Design review of the part built by this model. Coordinates are the model's own, in mm. Face numbers are marked on the shaded views. A direction names the side the tool comes from. Round coordinates to 2 decimals unless told otherwise and drop trailing zeros. Loops run counter-clockwise (first coordinate to the right, second up) from the corner with the lowest first, then second, coordinate; pieces in that order, holes last. Notation, with made-up numbers: (-14.75, 53.25) -> (32.25, 53.25) arc R27 cw to (32.25, 77.25) -> close; hole circle Ø1 at (-31, 27). An arc over 180 degrees is marked (long way). Answer as CSV lines item,"result". Start each with the question number.
```python
from build123d import *

# Parameters (mm, degrees)
F1_DEPTH = 10
F2_W     = 30
F2_H     = 30
F3_DEPTH = 28.5
F4_R     = 10.5
F5_DEPTH = 57.001


with BuildPart() as f1:
    # F0 (on Top) → F1 (new body, symmetric)
    with BuildSketch(Plane.XY):
        Polygon((-12.5, -25), (12.5, -25), (12.5, 25), (-12.5, 25), (-12.5, 15), (-54.5, 15), (-54.5, -15), (-12.5, -15), align=None)
    extrude(amount=F1_DEPTH, both=True)

    # F2 (on Top) → F3 (join, symmetric)
    with BuildSketch(Plane.XY):
        with Locations((-39.5, 0)):
            Rectangle(F2_W, F2_H)
    extrude(amount=F3_DEPTH, both=True)

    # F4 (on face) → F5 (cut, through all)
    with BuildSketch(Plane.XY.offset(28.5)):
        with Locations((-39.5, 0)):
            Circle(F4_R)
    extrude(amount=-F5_DEPTH, mode=Mode.SUBTRACT)


solid = f1.part
```
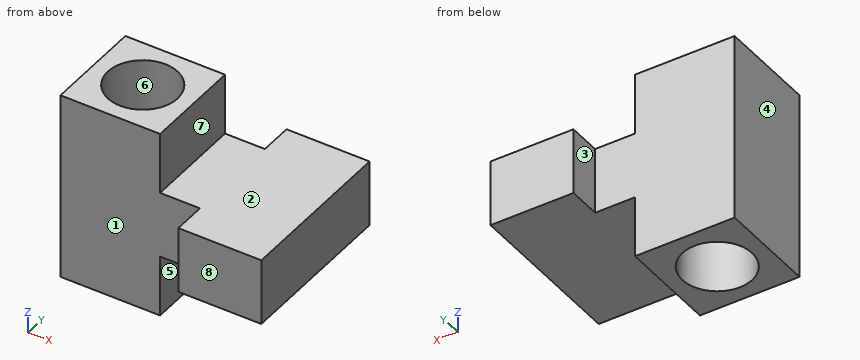
Q1. Add section A-A, the plane y = 0. Give the boundary of the cut face in (x, z).
Q2. Mouldability with a two-part tool opening along X and no side actions: class the marked faces 6, 7 and 8 as pulls with the +X half, pulls with the -X half, needs draft (parallel to the pull), parting line crosses it, or undercut.
Q3. Machinability: for the marked faces 1, 2, 3, 4 and 5, which of the approach directions +Z, -Z, +X, -X, +Y, -Y give a long, thin tool a straight path to every point of the face, cutting with its end or side? Answer none if there is none.
Q4. Add section C-C, the plane z = -7. Give the boundary of the cut face in (x, y).
Q5. For pin 1 Ø12 at (x, z) = (-41, 8) entering from +Y; pin 2 Ø5 at (x, z) = (-42, 16.5) entering from -Y; pin 3 Ø8 at (y, z) = (-20.5, 0.5) entering from -X, all flat-tipped, find the tip position at first contact; note any pin that passes through.
Q6. Add section D-D, the plane y = -5. Give the boundary of the cut face in (x, z), and give its area (3 significant figures).
Q7. To check wall thickness, follow probe 1 along Y at (x, z) = (-39.5, 12.5); probe 2 along Z at (x, y) = (-4.5, -4); probe 3 along Y at (x, z) = (-19, -3). State the ranges of each line that lie inside material, in increasing order. Write a range as from..to.
Q8. Add section B-B, the plane x = -39.5. Give the boundary of the cut face in (y, z).
Worked answers:
1,outline,"(-54.5, -28.5) -> (-50, -28.5) -> (-50, 28.5) -> (-54.5, 28.5) -> close; (-29, -28.5) -> (-24.5, -28.5) -> (-24.5, -10) -> (12.5, -10) -> (12.5, 10) -> (-24.5, 10) -> (-24.5, 28.5) -> (-29, 28.5) -> close"
2,face 6,"undercut"
2,face 7,"pulls with the +X half"
2,face 8,"needs draft"
3,face 1,"+Z, -Z, -X, -Y"
3,face 2,"+Z, +X, +Y, -Y"
3,face 3,"+Z, -Z, -X, +Y"
3,face 4,"+Z, -Z, -X, +Y, -Y"
3,face 5,"-Z, +X, +Y, -Y"
4,outline,"(-54.5, -15) -> (-12.5, -15) -> (-12.5, -25) -> (12.5, -25) -> (12.5, 25) -> (-12.5, 25) -> (-12.5, 15) -> (-54.5, 15) -> close; hole circle Ø21 at (-39.5, 0)"
5,pin 1,"stops at y = 15"
5,pin 2,"stops at y = -15"
5,pin 3,"stops at x = -12.5"
6,outline,"(-54.5, -28.5) -> (-48.73, -28.5) -> (-48.73, 28.5) -> (-54.5, 28.5) -> close; (-30.27, -28.5) -> (-24.5, -28.5) -> (-24.5, -10) -> (12.5, -10) -> (12.5, 10) -> (-24.5, 10) -> (-24.5, 28.5) -> (-30.27, 28.5) -> close"
6,area,"1,400 mm^2"
7,probe 1,"y = -15..-10.5, 10.5..15"
7,probe 2,"z = -10..10"
7,probe 3,"y = -15..15"
8,outline,"(-15, -28.5) -> (-10.5, -28.5) -> (-10.5, 28.5) -> (-15, 28.5) -> close; (10.5, -28.5) -> (15, -28.5) -> (15, 28.5) -> (10.5, 28.5) -> close"
